Check sheet for the modelled part. Datum: model origin and axes. Units: mm. A direction names the side the tool comes from. Round coordinates to 2 decimals unless told otherwise and drop trailing zeros. Order: outer loops, then holes, each group sorted by start corner. A loop starts at its lowest first (then second) coordinate and runs counter-clockwise, first axis right, second up. Notation, with made-up numbers: (-21.5, 51) -> (2.5, 51) arc R20 cw to (2.5, 82) -> close; hole circle Ø9 at (3.25, -32.75). An arc over 180 degrees is marked (long way). Answer as CSV lines item,"result". Start each with the question number.
from build123d import *

# Parameters (mm, degrees)
SKETCH_W                  = 37.3126
SKETCH_H                  = 69.215
CORE_HOLDER_PLATE_F_DEPTH = 3.175
F_8_CLEARANCE_HOLE2_D     = 4.4958


with BuildPart() as part:
    # Sketch → CORE_HOLDER_PLATE-F (new body)
    with BuildSketch(Plane(origin=(0, 35.89274, 0), x_dir=(1, 0, 0), z_dir=(0, 1, 0))):
        with BuildLine():
            Line((7.6454, 69.85), (7.6454, -69.85))
            ThreePointArc((7.6454, -69.85), (0, -77.4954), (-7.6454, -69.85))
            Line((-7.6454, -69.85), (-7.6454, 69.85))
            ThreePointArc((-7.6454, 69.85), (0, 77.4954), (7.6454, 69.85))
        make_face()
        with Locations((26.3017, 0)):
            Rectangle(SKETCH_W, SKETCH_H)
    extrude(amount=CORE_HOLDER_PLATE_F_DEPTH)

    # #8 Clearance Hole2 (through all)
    with Locations(Plane.XZ.offset(-35.89274)):
        with Locations((0, 69.85), (0, -69.85)):
            Hole(F_8_CLEARANCE_HOLE2_D / 2)


solid = part.part
1) Section check A-A on x = 0. Record the cut outline in (y, z).
2) Material ranges on line 1 along Z through (x, y) = (0, 36.65); line 2 along Z through (x, y) = (28, 36); line 3 along X through (y, z) = (37.3, 46), recorded low to high.
3) Section check D-D on z = 44. Record the cut outline in (x, y).
4) Access from +Z, -Z, +X, -X, +Y, -Y to the whole of each face (thin tool, end or side, straight path). Record for faces 1 (the face through (26, 37, -34.608)), 2 (the face through (26, 37, 34.608)), 3 (the face through (13, 35.893, -1)).
5) Section check C-C on x = 35. Record the cut outline in (y, z), then the cut area to 3 significant figures.
6) Section check B-B on y = 36.75. Record the cut outline in (x, z).
7) Depth check by flat-ended pin: pin 1 Ø1.6 at (x, y) = (29.5, 37.5) entering from +Z; pin 2 Ø1.6 at (x, y) = (19.5, 37) entering from -Z; pin 3 Ø1.6 at (y, z) = (37.5, -51) entering from +X. Enter the tip coordinate at first touch or a pass-through.
Solutions:
1,outline,"(35.89, -77.5) -> (39.07, -77.5) -> (39.07, -72.1) -> (35.89, -72.1) -> close; (35.89, -67.6) -> (39.07, -67.6) -> (39.07, 67.6) -> (35.89, 67.6) -> close; (35.89, 72.1) -> (39.07, 72.1) -> (39.07, 77.5) -> (35.89, 77.5) -> close"
2,line 1,"z = -77.5 to -72.1, -67.6 to 67.6, 72.1 to 77.5"
2,line 2,"z = -34.61 to 34.61"
2,line 3,"x = -7.65 to 7.65"
3,outline,"(-7.65, 35.89) -> (7.65, 35.89) -> (7.65, 39.07) -> (-7.65, 39.07) -> close"
4,face 1,"-Z, +X, +Y, -Y"
4,face 2,"+Z, +X, +Y, -Y"
4,face 3,"+Z, -Z, +X, -X, -Y"
5,outline,"(35.89, -34.61) -> (39.07, -34.61) -> (39.07, 34.61) -> (35.89, 34.61) -> close"
5,area,"220 mm^2"
6,outline,"(-7.65, -69.85) arc R7.65 ccw to (7.65, -69.85) -> (7.65, -34.61) -> (44.96, -34.61) -> (44.96, 34.61) -> (7.65, 34.61) -> (7.65, 69.85) arc R7.65 ccw to (-7.65, 69.85) -> close; hole circle Ø4.5 at (0, -69.85); hole circle Ø4.5 at (0, 69.85)"
7,pin 1,"stops at z = 34.61"
7,pin 2,"stops at z = -34.61"
7,pin 3,"stops at x = 7.65"
